from build123d import *

# Parameters (mm, degrees)
F0_R     = 2.01
F0_R_2   = 7.5
F1_DEPTH = 5
F2_R     = 11.01
F3_DEPTH = 3
F4_R     = 17.5
F4_R_2   = 11.01
F5_DEPTH = 4.2
F6_SIZE  = 4.19999
F7_SIZE  = 3


# Not quite as in the source:
# - a fillet or chamfer is up to 0.001 mm smaller than in the source, because OpenCascade refuses the exact size


with BuildPart() as f1:
    # F0 (on Front) → F1 (new body)
    with BuildSketch(Plane.XZ):
        Polygon((0, 80), (0, 0), (65, 0), (80, 15), (80, 80), align=None)
        with Locations((10, 10)):
            Circle(F0_R, mode=Mode.SUBTRACT)
        with Locations((58.25, 35)):
            Circle(F0_R_2, mode=Mode.SUBTRACT)
        with Locations((10, 40)):
            Circle(F0_R, mode=Mode.SUBTRACT)
        with Locations((10, 70)):
            Circle(F0_R, mode=Mode.SUBTRACT)
        with Locations((40, 70)):
            Circle(F0_R, mode=Mode.SUBTRACT)
        with Locations((70, 70)):
            Circle(F0_R, mode=Mode.SUBTRACT)
    extrude(amount=F1_DEPTH)

    # F2 (on face) → F3 (cut)
    with BuildSketch(Plane.XZ.offset(5)):
        with Locations((58.25, 35)):
            Circle(F2_R)
    extrude(amount=-F3_DEPTH, mode=Mode.SUBTRACT)

    # F4 (on face) → F5 (join)
    with BuildSketch(Plane.XZ.offset(5)):
        with Locations((58.25, 35)):
            Circle(F4_R)
        with Locations((58.25, 35)):
            Circle(F4_R_2, mode=Mode.SUBTRACT)
    extrude(amount=F5_DEPTH)

    # F6 (size 4.2 in the source; OpenCascade refuses exactly that, so slightly less here)
    f6_edges = [f1.edges().sort_by_distance(p)[0] for p in [
        (40.75, -9.2, 35),
    ]]
    chamfer(f6_edges, length=F6_SIZE)

    # F7
    f7_edges = [f1.edges().sort_by_distance(p)[0] for p in [
        (40, 0, 80),
        (80, 0, 47.5),
        (72.5, 0, 7.5),
        (0, 0, 40),
        (32.5, 0, 0),
    ]]
    chamfer(f7_edges, length=F7_SIZE)


with BuildPart() as f8_1:
    # F8: copy of F1
    add(f1.part)


solid = f1.part
Model file for the job. Use its own axes, mm. A direction names the side the tool comes from. Give positions to 0.01 mm unless a question says otherwise; leave off trailing zeros. Loops run counter-clockwise (first coordinate to the right, second up) from the corner with the lowest first, then second, coordinate; pieces in that order, holes last. Notation, with made-up numbers: (30, 26.25) -> (62, 26.25) arc R35 ccw to (62, 58.25) -> close; hole circle Ø6 at (-7.5, -23.75). An arc over 180 degrees is marked (long way). Use a Markdown table: item, result. Add a question column.
(1) Tool access for faces 1 (the flat face through (55.6, -2, 27.8)), 2 (the flat face through (71.32, -1.48, 8.47)): list every direction of +Z, -Z, +X, -X, +Y, -Y with a clear straight run to the whole face (end or side of a thin tool).
(2) Slice it at D-D on x = 34.5. List the corners of the cut face in (y, z).
(3) Slice it at A-A on z = 70. List the corners of the cut face in (x, y).
(4) Wall check: line 1 along Y through (x, z) = (24, 67); line 2 along X through (y, z) = (-0.6, 35); line 3 along Z through (x, y) = (70, -3.2). Give the ranges that are in metal, low to high.
(5) Drop flat-ended pins along their axis: pin 1 Ø1.5 at (x, z) = (66, 40) entering from -Y; pin 2 Ø17 at (x, z) = (58.25, 35) entering from +Y; pin 3 Ø5 at (x, z) = (10, 70) entering from -Y; pin 4 Ø4 at (x, y) = (18, -7.5) entering from -Z. Give the stop position or say it passes through.
Filled sheet:
| question | item | result |
|---|---|---|
| 1 | face 1 | -Y |
| 1 | face 2 | -Z, +X, +Y |
| 2 | outline | (-5, 0) -> (-3, 0) -> (0, 3) -> (0, 77) -> (-3, 80) -> (-5, 80) -> close |
| 3 | outline | (0, -5) -> (7.99, -5) -> (7.99, 0) -> (3, 0) -> (0, -3) -> close; (12.01, -5) -> (37.99, -5) -> (37.99, 0) -> (12.01, 0) -> close; (42.01, -5) -> (67.99, -5) -> (67.99, 0) -> (42.01, 0) -> close; (72.01, -5) -> (80, -5) -> (80, -3) -> (77, 0) -> (72.01, 0) -> close |
| 4 | line 1 | -5 to 0 |
| 4 | line 2 | 2.4 to 50.75, 65.75 to 77.6 |
| 4 | line 3 | 5 to 67.99, 72.01 to 80 |
| 5 | pin 1 | y = -2 |
| 5 | pin 2 | y = 0 |
| 5 | pin 3 | y = -5 |
| 5 | pin 4 | through |
